Check sheet for the drawn part. Datum: minimum x, y, z corner. Units: mm. A direction names the side the tool comes from. Coordinates: 2 decimals unless noted, no trailing zeros. Write each loop counter-clockwise with the first axis right and the second up, starting at its lowest first coordinate (ties: lowest second). Pieces come first, ordered by that corner, then holes. Notation, with made-up numbers: (82.5, 67.25) -> (129.5, 67.25) arc R24 cw to (129.5, 103.25) -> close; hole circle Ø3 at (-33.75, 64.5). An arc over 180 degrees is marked (long way). Answer in a Markdown table with one row per item. Add a question column.
Q1. Gauge pin test, flat ends, axial feed: P1, Ø0.5, axis at x = 28, z = 16, coming from the +Y side; P2, Ø1.1, axis at y = 9, z = 0.5, coming from the +X side; P3, Ø4.5, axis at x = 14.5, z = 10, coming from the +Y side. Record the tip position at first contact, or that the pin passes through.
Q2. Release check for a two-part mould opening along Z. For the marked faces 3, 4 and 5 record: pulls with the +Z half, pulls with the -Z half, needs draft (parallel to the pull), parting line crosses it, or undercut.
Q3. Section check D-D, the plane x = 22.5. Record the boundary of the cut face in (y, z).
Q4. Tool access check on the marked faces 1 and 2. Record the directions out of +Z, -Z, +X, -X, +Y, -Y that give a thin tool (end or side, any length) a straight path to the whole face; none if there is none.
Q5. Section check A-A, the plane x = 39. Record the boundary of the cut face in (y, z).
Q6. Thickness scan on line 1 (X direction, y = 11, z = 6.25); line 2 (Z direction, x = 19.5, y = 9.5); line 3 (Y direction, x = 12, z = 5.5). Record the ranges inside material, lowest first.
Q7. Section check B-B, the plane y = 32. Record the boundary of the cut face in (x, z).
Q8. Section check C-C, the plane y = 16. Record the boundary of the cut face in (x, z).
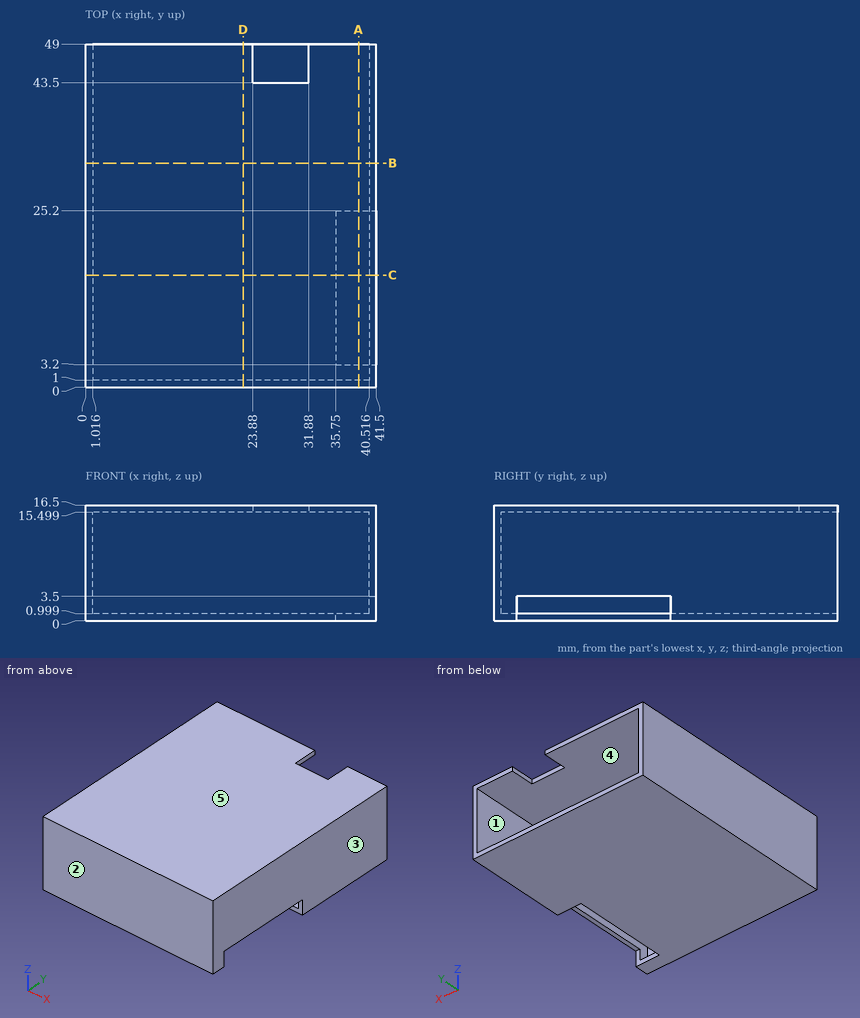
Calculated:
| question | item | result |
|---|---|---|
| 1 | P1 | stops at y = 43.5 |
| 1 | P2 | stops at x = 35.75 |
| 1 | P3 | stops at y = 1 |
| 2 | face 3 | needs draft |
| 2 | face 4 | undercut |
| 2 | face 5 | pulls with the +Z half |
| 3 | outline | (0, 0) -> (49, 0) -> (49, 1) -> (1, 1) -> (1, 15.5) -> (49, 15.5) -> (49, 16.5) -> (0, 16.5) -> close |
| 4 | face 1 | +Y |
| 4 | face 2 | +Z, -Z, +X, -X, -Y |
| 5 | outline | (0, 0) -> (3.2, 0) -> (3.2, 1) -> (1, 1) -> (1, 15.5) -> (49, 15.5) -> (49, 16.5) -> (0, 16.5) -> close; (25.2, 0) -> (49, 0) -> (49, 1) -> (25.2, 1) -> close |
| 6 | line 1 | x = 0 to 1.02, 40.52 to 41.5 |
| 6 | line 2 | z = 0 to 1, 15.5 to 16.5 |
| 6 | line 3 | y = 0 to 1 |
| 7 | outline | (0, 0) -> (41.5, 0) -> (41.5, 16.5) -> (0, 16.5) -> close; hole (1.02, 1) -> (40.52, 1) -> (40.52, 15.5) -> (1.02, 15.5) -> close |
| 8 | outline | (0, 0) -> (35.75, 0) -> (35.75, 1) -> (1.02, 1) -> (1.02, 15.5) -> (40.52, 15.5) -> (40.52, 3.5) -> (41.5, 3.5) -> (41.5, 16.5) -> (0, 16.5) -> close |
